Build history of the part. All positions in model axes, mm. Coordinates: 2 decimals unless noted, no trailing zeros. Order: outer loops, then holes, each group sorted by start corner. A loop starts at its lowest first (then second) coordinate and runs counter-clockwise, first axis right, second up. Notation, with made-up numbers: (24.25, 8.25) - (43.25, 8.25) arc R22 ccw to (43.25, 28.25) - close; hole circle Ø7 at (51, 69). An arc over 180 degrees is marked (long way). One line per item, written item: value.
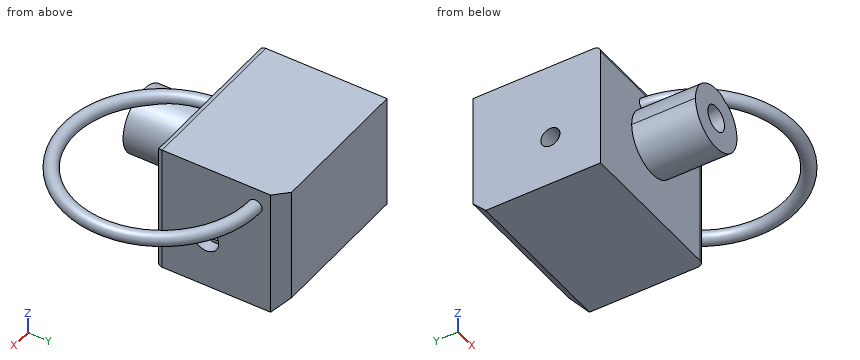
Autodesk Inventor part; units mm, degrees
ref_plane "YZ Plane" through (0, 0, 0) normal (1, 0, 0) x (0, 1, 0)
ref_plane "XZ Plane" through (0, 0, 0) normal (0, 1, 0) x (-1, 0, 0)
ref_plane "XY Plane" through (0, 0, 0) normal (0, 0, 1) x (1, 0, 0)
sketch "Szkic1" plane through (0, 0, 0) normal (0, 1, 0) x (-1, 0, 0)
  circle A0 centre (0, 0) radius 5
  circle A1 centre (0, 0) radius 2
  dimension "d0" = 10
  dimension "d1" = 3
extrude "Wyciągnięcie proste1" add sketch "Szkic1" along normal blind 10
sketch "Szkic2" plane through (0, 10, 0) normal (0, 1, 0) x (1, 0, 0)
  circle A0 centre (0, 0) radius 5
  circle A1 centre (0, 0) radius 2
  line L0 (-12.5, 11.7523) -> (12.5, 11.7523)
  line L1 (12.5, 11.7523) -> (12.5, -8.2477)
  line L2 (12.5, -8.2477) -> (-12.5, -8.2477)
  line L3 (-12.5, -8.2477) -> (-12.5, 11.7523)
  line L4 (0, 11.1673) -> (0, -8.4509) construction
  dimension "d4" = 20
  dimension "d5" = 25
extrude "Wyciągnięcie proste2" add sketch "Szkic2" along normal blind 20 contours A0 | A1 | L0 L1 L2 L3
fillet "Zaokrąglenie1" radius 1 2 edges at (0, 10, 8.2477) (12.5, 10, -1.7523)
chamfer "Faza1" distance 2 angle 45 2 edges at (12.5, 30, -1.7523) (0, 30, -11.7523)
sketch "Szkic3" plane through (12.5, 11, 8.2477) normal (1, 0, 0) x (0, 0, -1)
  line L0 (0, 17) -> (20, 17)
  line L1 (0, 0) -> (0, 17)
  line L2 (20, 0) -> (0, 0)
  line L3 (20, 0) -> (20, 17)
  circle A0 centre (2.9885, 14.5933) radius 1.0701
  line L4 (9.4628, 11.1568) -> (9.4628, 6.3913)
  line L5 (7.1085, 8.774) -> (15.0257, 8.774)
  point P0 (8.2477, -11)
revolve "Obrót1" add sketch "Szkic3" angle 360 about axis through (12.5, 11, -11.7523) along (0, 0, 1) contours A0
sketch "Szkic4" plane through (12.5, 11, 8.2477) normal (1, 0, 0) x (0, 0, -1)
  point P0 (8.2477, -11)
  point P1 (12.057, 6.8711)
hole "Otwór1" at (12.5, 17.8711, -3.8093) direction (-1, 0, 0) diameter 3 end through all counterbore diameter 4 counterbore depth 2
1. Band-saw the part on D-D, the plane z = 3.5. Give the cut face in (x, y), and give its area (3 significant figures).
Values found:
outline: (-12.5, 10) - (-3.57, 10) - (-3.57, 0) - (3.57, 0) - (3.57, 10) - (11.5, 10) arc R1 ccw to (12.5, 11) - (12.5, 28) - (10.5, 30) - (-12.5, 30) - close
area: 569 mm2
2. Probe line 1 along X through (y, z) = (18, -0.25); line 2 along Y through (x, z) = (-7.5, -1.5); line 3 along Z through (x, y) = (-0.5, 6.5). List the from-to ranges inside material, lowest first.
Values found:
line 1: x = -12.5 to 12.5
line 2: y = 10 to 30
line 3: z = -4.97 to -1.94, 1.94 to 5.93
3. Band-saw the part on B-B, the plane x = 6. Count the separate pieces of the cut face and the enclosed holes in it, and give its area (3 significant figures).
Values found:
separate pieces: 2
enclosed holes: 1
area: 395 mm2
4. Band-saw the part on A-A, the plane z = -8. Give the cut face in (x, y).
Values found:
outline: (-12.5, 10) - (11.5, 10) arc R1 ccw to (12.5, 11) - (12.5, 28) - (10.5, 30) - (-12.5, 30) - close
5. Flat gauge pins, fed straight in: P1, Ø5, axis at x = 0, z = 0, coming from the -Y side; P2, Ø8, axis at y = 0, z = 6, coming from the -X side; P3, Ø10, axis at y = 1, z = 2, coming from the +X side; P4, Ø6.5, axis at y = 17.87, z = -3.81, coming from the -X side. Where does each tip first touch, or does it go through?
Values found:
P1: stops at y = 0
P2: stops at x = -4.58
P3: stops at x = 26.93
P4: stops at x = -12.5
